Study the drawing (mm; zero at the part's minimum x, y, z) and answer. A direction names the side the tool comes from. Round coordinates to 2 decimals unless told otherwise and drop trailing zeros. Loops run counter-clockwise (first coordinate to the right, second up) from the corner with the lowest first, then second, coordinate; pieces in that order, holes last. Notation, with made-up numbers: (-6, 47.25) -> (34, 47.25) arc R28 cw to (34, 65.25) -> close; hole circle Ø3 at (25.25, 22). An arc over 180 degrees is marked (long way). Write each question's results on one line, items separated by ' | '. Start each with the question number.
(1) The part is cut by section A-A (z = 3.5). Determine the outline of the cut face in (x, y).
(2) Straight lines are drawn through the part: probe 1 along X at (y, z) = (4.5, 3.9); probe 2 along Y at (x, z) = (14.5, 4.6). For each, find the intervals that lie inside material, in ascending order.
(3) Flat-ended cylindrical pins translate along their axes: pin 1 (1.5 mm diameter, centred on x = 17, y = 41.5, fed in from -Z); pin 2 (1.5 mm diameter, centred on y = 2, z = 3, fed in from -X); pin 3 (2.5 mm diameter, centred on y = 88.5, z = 2.5, fed in from +X); pin 4 (2.5 mm diameter, centred on x = 25, z = 2, fed in from +Y). Find the tip coordinate at first contact, or state that the pin passes through.
(4) For the marked faces 1, 2 and 3, determine the directions among +Z, -Z, +X, -X, +Y, -Y from which every point of the face is accessible in a straight line to the end or side of a thin tool.
(5) The part is cut by section B-B (x = 2). Determine the outline of the cut face in (y, z).
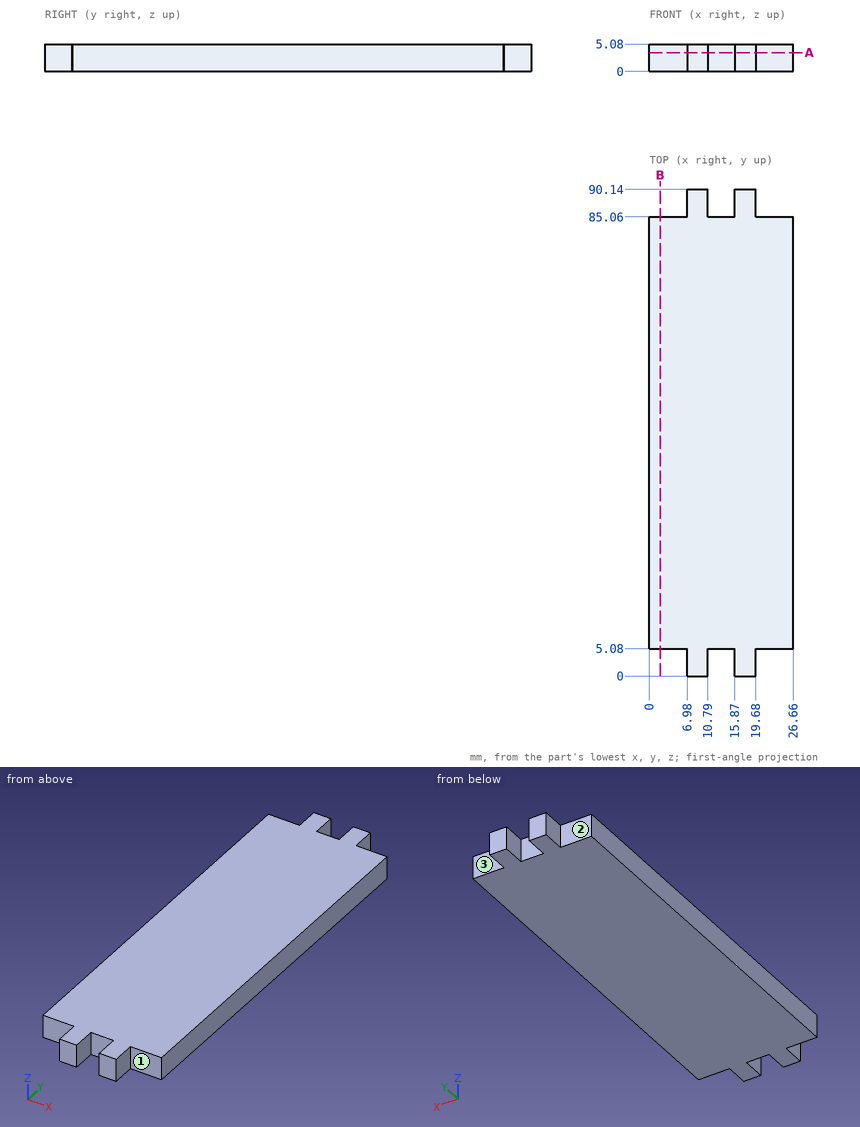
Checked values:
1) outline: (0, 5.08) -> (6.98, 5.08) -> (6.98, 0) -> (10.79, 0) -> (10.79, 5.08) -> (15.87, 5.08) -> (15.87, 0) -> (19.68, 0) -> (19.68, 5.08) -> (26.66, 5.08) -> (26.66, 85.06) -> (19.68, 85.06) -> (19.68, 90.14) -> (15.87, 90.14) -> (15.87, 85.06) -> (10.79, 85.06) -> (10.79, 90.14) -> (6.98, 90.14) -> (6.98, 85.06) -> (0, 85.06) -> close
2) probe 1: x = 6.98 to 10.79, 15.87 to 19.68 | probe 2: y = 5.08 to 85.06
3) pin 1: stops at z = 0 | pin 2: stops at x = 6.98 | pin 3: stops at x = 19.68 | pin 4: stops at y = 85.06
4) face 1: +Z, -Z, +X, -Y | face 2: +Z, -Z, -X, +Y | face 3: +Z, -Z, +X, +Y
5) outline: (5.08, 0) -> (85.06, 0) -> (85.06, 5.08) -> (5.08, 5.08) -> close
